Drawing for the job (mm, zero at the part's lowest x, y, z). A direction names the side the tool comes from. Give positions to 0.01 mm unless a question says otherwise; leave off trailing zeros. Order: outer loops, then holes, each group sorted by start corner. A loop starts at its lowest first (then second) coordinate and runs counter-clockwise, first axis right, second up. Notation, with made-up numbers: (38, 57) - (79, 57) arc R31 cw to (79, 96) - close; hole circle Ø4 at (-1.75, 41). An arc over 180 degrees is marked (long way). One line per item, written item: value.
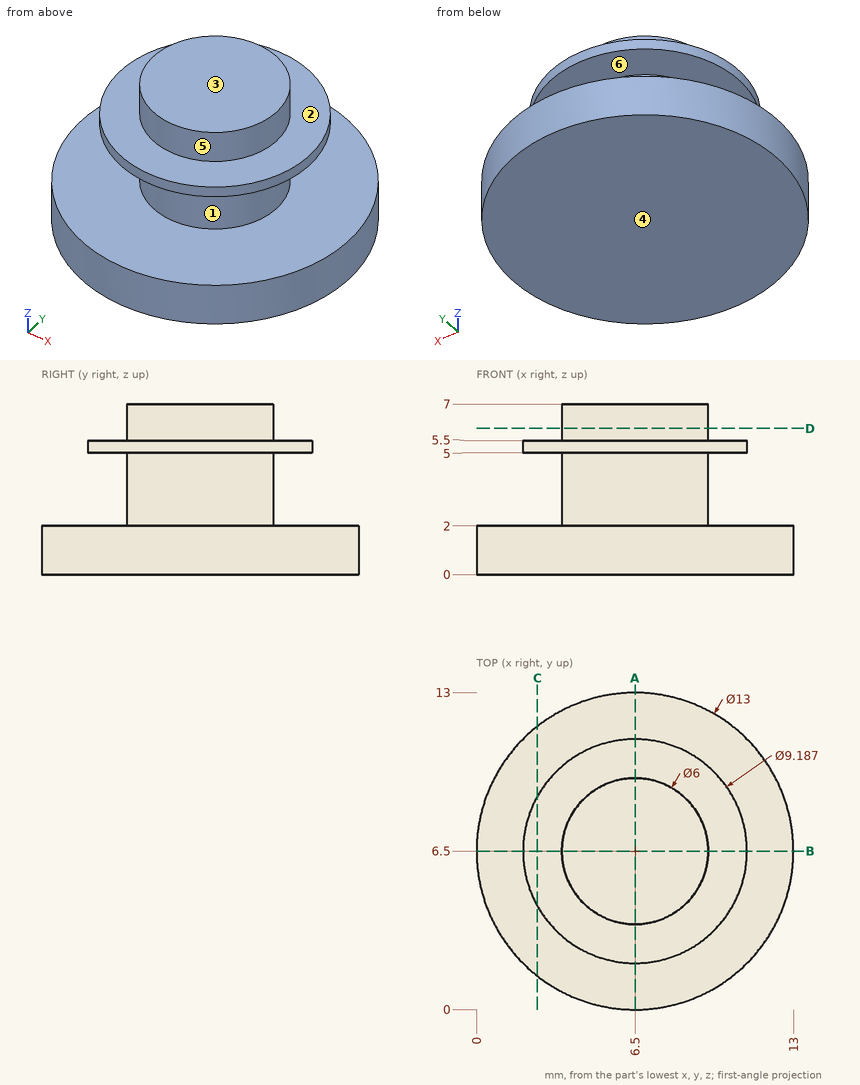
(1) Pull direction Z, two halves, no side cores. Call the marked faces 4, 5 and 6: +Z half, -Z half, draft (parallel to the pull), parting line (faces both ways), or undercut.
Completed:
face 4: -Z half
face 5: draft
face 6: undercut
(2) Pin check, flat tip, straight feed: P1, Ø4, axis at x = 11, z = 2.5, coming from the -Y side. Stop position of the tip, or through.
Completed:
P1: y = 0.53
(3) Slice it at C-C, the plane x = 2.5. Give the cut face in (y, z).
Completed:
outline: (1.38, 0) - (11.62, 0) - (11.62, 2) - (1.38, 2) - close; (4.24, 5) - (8.76, 5) - (8.76, 5.5) - (4.24, 5.5) - close
(4) Drill centre lines: line 1 (Z direction, x = 7.75, y = 3.25); line 2 (Z direction, x = 2, y = 8.25); line 3 (Y direction, x = 3.5, z = 1.5). Where is each one in solid material? Low to high.
Completed:
line 1: 0 to 2, 5 to 5.5
line 2: 0 to 2
line 3: 0.73 to 12.27
(5) Slice it at D-D, the plane z = 6. Give the cut face in (x, y), and give its area (3 significant figures).
Completed:
outline: circle Ø6 at (6.5, 6.5)
area: 28.3 mm²
(6) Slice it at A-A, the plane x = 6.5. Give the cut face in (y, z), and give its area (3 significant figures).
Completed:
outline: (0, 0) - (13, 0) - (13, 2) - (9.5, 2) - (9.5, 5) - (11.09, 5) - (11.09, 5.5) - (9.5, 5.5) - (9.5, 7) - (3.5, 7) - (3.5, 5.5) - (1.91, 5.5) - (1.91, 5) - (3.5, 5) - (3.5, 2) - (0, 2) - close
area: 57.6 mm²
(7) 3-axis set-ups, long thin cutter, end or side, ignore diameter. For the marked faces 1, 2 and 3: which of +Z, -Z, +X, -X, +Y, -Y reach the whole face in a straight line?
Completed:
face 1: none
face 2: +Z
face 3: +Z, +X, -X, +Y, -Y
